Can you work these out from the model? Positions are in its coordinate system, mm. A direction names the side the tool comes from. Give positions to 0.01 mm unless a question says otherwise; leave off trailing zeros. Write each loop counter-clockwise with the first axis right and the second up, starting at its lowest first coordinate (ties: lowest second). Pieces come first, ordered by that corner, then holes. Notation, with made-up numbers: M 7,4 L 43,4 A13 ccw 43,14 Z; hole C 85.5,-14 d4. An arc over 180 degrees is marked long. Write each question's results on one line, items separated by ' | '.
from build123d import *

# Parameters (mm, degrees)
F1_DEPTH = 12.7


with BuildPart() as f1:
    # F0 (on Right) → F1 (new body)
    with BuildSketch(Plane.YZ):
        with BuildLine():
            Line((0, 41.94333), (0, 0))
            Line((0, 0), (73.158316, 0))
            Line((73.158316, 0), (73.158316, 41.94333))
            ThreePointArc((73.158316, 41.94333), (69.438572, 50.923586), (60.458316, 54.64333))
            Line((60.458316, 54.64333), (12.7, 54.64333))
            ThreePointArc((12.7, 54.64333), (3.719744, 50.923586), (0, 41.94333))
        make_face()
        with BuildLine():
            ThreePointArc((9.530765, 22.352), (11.837006, 27.919759), (17.404765, 30.226))
            Line((17.404765, 30.226), (55.504765, 30.226))
            ThreePointArc((55.504765, 30.226), (61.072524, 27.919759), (63.378765, 22.352))
            ThreePointArc((63.378765, 22.352), (61.072524, 16.784241), (55.504765, 14.478))
            Line((55.504765, 14.478), (17.404765, 14.478))
            ThreePointArc((17.404765, 14.478), (11.837006, 16.784241), (9.530765, 22.352))
        make_face(mode=Mode.SUBTRACT)
    extrude(amount=F1_DEPTH)


solid = f1.part
Item 1: Thinking about a two-plate mould opening in Y: for faces 1 (the face through (0, 36, 34)), 2 (the face through (6, 0, 21)), 3 (the face through (6, 73.158, 21)), 4 (the face through (6, 37, 14.478)), which applies, +Y half, -Y half, draft (parallel to the pull), parting line (faces both ways), or undercut?
Geometry says:
face 1: draft | face 2: -Y half | face 3: +Y half | face 4: undercut
Item 2: I want a section at C-C, the plane z = 28. Please give me the cut outline in (x, y).
Geometry says:
outline: M 0,0 L 12.7,0 L 12.7,11.92 L 0,11.92 Z; M 0,60.99 L 12.7,60.99 L 12.7,73.16 L 0,73.16 Z
Item 3: I want a section at B-B, the plane x = 11.25. Please give me the cut outline in (y, z).
Geometry says:
outline: M 0,0 L 73.16,0 L 73.16,41.94 A12.7 ccw 60.46,54.64 L 12.7,54.64 A12.7 ccw 0,41.94 Z; hole M 9.53,22.35 A7.87 ccw 17.4,14.48 L 55.5,14.48 A7.87 ccw 63.38,22.35 A7.87 ccw 55.5,30.23 L 17.4,30.23 A7.87 ccw Z
Item 4: I'm going to push flat-ended pins straight in: pin 1 (2 mm diameter, centred on y = 14, z = 31.5, fed in from -X); pin 2 (3 mm diameter, centred on x = 2, y = 11, fed in from +Z). Where does each tip first touch, or does it pass through?
Geometry says:
pin 1: stops at x = 0 | pin 2: stops at z = 54.64
Item 5: I want a section at D-D, the plane y = 6.5. Please give me the cut outline in (x, z), and give its area (3 significant figures).
Geometry says:
outline: M 0,0 L 12.7,0 L 12.7,53.03 L 0,53.03 Z | area: 673 mm2
Item 6: For faces 5 (the face through (6, 36, 0)), 6 (the face through (6, 36, 30.226)), which set-ups out of +Z, -Z, +X, -X, +Y, -Y let a thin tool reach every point of the face, with its end or its side?
Geometry says:
face 5: -Z, +X, -X, +Y, -Y | face 6: +X, -X
Item 7: If I drill on line 1 (Z direction, x = 8, y = 42); line 2 (Y direction, x = 11, z = 22.5); line 3 (Y direction, x = 10.5, z = 29), over which ranges is the centre line in solid material (lowest first)? Write a range as from..to.
Geometry says:
line 1: z = 0..14.48, 30.23..54.64 | line 2: y = 0..9.53, 63.38..73.16 | line 3: y = 0..13.19, 59.72..73.16
Item 8: I want a section at A-A, the plane y = 43.5. Please give me the cut outline in (x, z), and give its area (3 significant figures).
Geometry says:
outline: M 0,0 L 12.7,0 L 12.7,14.48 L 0,14.48 Z; M 0,30.23 L 12.7,30.23 L 12.7,54.64 L 0,54.64 Z | area: 494 mm2
